from build123d import *

# Parameters (mm, degrees)
SKETCH2_R               = 18
SKETCH2_W               = 7.5
SKETCH2_H               = 7.5
BOSS_EXTRUDE1_DEPTH     = 0.9
BOSS_EXTRUDE10_START    = 0.4
SKETCH18_W              = 7.7
SKETCH18_H              = 7.7
BOSS_EXTRUDE10_DEPTH    = 0.4
BOSS_EXTRUDE2_START     = -1
SKETCH3_R               = 35
SKETCH3_R_2             = 18
BOSS_EXTRUDE2_DEPTH     = 1
SKETCH4_R               = 2.9
BOSS_EXTRUDE3_DEPTH     = 3
CUT_EXTRUDE1_DEPTH      = 50.588305073
CUT_EXTRUDE1_DEPTH_BACK = 50.588305073
SKETCH7_R               = 59.131365533
FILLET1_R               = 6


with BuildPart() as part:
    # Sketch2 → Boss-Extrude1 (new body)
    with BuildSketch(Plane.XY.offset(10)):
        Circle(SKETCH2_R)
        with BuildLine():
            Line((-8.15, -8.35), (-8.15, -14.91903147))
            ThreePointArc((-8.15, -14.91903147), (-11.939670478, -12.101415986), (-14.808021475, -8.35))
            Line((-14.808021475, -8.35), (-8.15, -8.35))
        make_face(mode=Mode.SUBTRACT)
        with BuildLine():
            Line((-8.15, -7.85), (-15.079041747, -7.85))
            ThreePointArc((-15.079041747, -7.85), (-16.470304718, -4.210589327), (-16.996396677, -0.35))
            Line((-16.996396677, -0.35), (-8.15, -0.35))
            Line((-8.15, -0.35), (-8.15, -7.85))
        make_face(mode=Mode.SUBTRACT)
        with BuildLine():
            Line((-8.15, 0.15), (-16.999338222, 0.15))
            ThreePointArc((-16.999338222, 0.15), (-16.521617742, 4.00451585), (-15.181485435, 7.65))
            Line((-15.181485435, 7.65), (-8.15, 7.65))
            Line((-8.15, 7.65), (-8.15, 0.15))
        make_face(mode=Mode.SUBTRACT)
        with BuildLine():
            Line((-8.15, 8.15), (-14.91903147, 8.15))
            ThreePointArc((-14.91903147, 8.15), (-12.02081528, 12.02081528), (-8.15, 14.91903147))
            Line((-8.15, 14.91903147), (-8.15, 8.15))
        make_face(mode=Mode.SUBTRACT)
        with BuildLine():
            Line((-7.65, 8.15), (-7.65, 15.181485435))
            ThreePointArc((-7.65, 15.181485435), (-4.00451585, 16.521617742), (-0.15, 16.999338222))
            Line((-0.15, 16.999338222), (-0.15, 8.15))
            Line((-0.15, 8.15), (-7.65, 8.15))
        make_face(mode=Mode.SUBTRACT)
        with BuildLine():
            Line((0.35, 8.15), (0.35, 16.996396677))
            ThreePointArc((0.35, 16.996396677), (4.210589327, 16.470304718), (7.85, 15.079041747))
            Line((7.85, 15.079041747), (7.85, 8.15))
            Line((7.85, 8.15), (0.35, 8.15))
        make_face(mode=Mode.SUBTRACT)
        with BuildLine():
            Line((8.35, 8.15), (8.35, 14.808021475))
            ThreePointArc((8.35, 14.808021475), (12.101415986, 11.939670478), (14.91903147, 8.15))
            Line((14.91903147, 8.15), (8.35, 8.15))
        make_face(mode=Mode.SUBTRACT)
        with BuildLine():
            Line((8.35, 7.65), (15.181485435, 7.65))
            ThreePointArc((15.181485435, 7.65), (16.521617742, 4.00451585), (16.999338222, 0.15))
            Line((16.999338222, 0.15), (8.35, 0.15))
            Line((8.35, 0.15), (8.35, 7.65))
        make_face(mode=Mode.SUBTRACT)
        with BuildLine():
            Line((8.35, -0.35), (16.996396677, -0.35))
            ThreePointArc((16.996396677, -0.35), (16.470304718, -4.210589327), (15.079041747, -7.85))
            Line((15.079041747, -7.85), (8.35, -7.85))
            Line((8.35, -7.85), (8.35, -0.35))
        make_face(mode=Mode.SUBTRACT)
        with BuildLine():
            Line((8.35, -8.35), (14.808021475, -8.35))
            ThreePointArc((14.808021475, -8.35), (12.02081528, -12.02081528), (8.35, -14.808021475))
            Line((8.35, -14.808021475), (8.35, -8.35))
        make_face(mode=Mode.SUBTRACT)
        with BuildLine():
            Line((7.85, -8.35), (7.85, -15.079041747))
            ThreePointArc((7.85, -15.079041747), (4.210589327, -16.470304718), (0.35, -16.996396677))
            Line((0.35, -16.996396677), (0.35, -8.35))
            Line((0.35, -8.35), (7.85, -8.35))
        make_face(mode=Mode.SUBTRACT)
        with BuildLine():
            Line((-0.15, -8.35), (-0.15, -16.999338222))
            ThreePointArc((-0.15, -16.999338222), (-4.00451585, -16.521617742), (-7.65, -15.181485435))
            Line((-7.65, -15.181485435), (-7.65, -8.35))
            Line((-7.65, -8.35), (-0.15, -8.35))
        make_face(mode=Mode.SUBTRACT)
        with Locations((-3.9, -4.1)):
            Rectangle(SKETCH2_W, SKETCH2_H, mode=Mode.SUBTRACT)
        with Locations((4.1, -4.1)):
            Rectangle(SKETCH2_W, SKETCH2_H, mode=Mode.SUBTRACT)
        with Locations((-3.9, 3.9)):
            Rectangle(SKETCH2_W, SKETCH2_H, mode=Mode.SUBTRACT)
        with Locations((4.1, 3.9)):
            Rectangle(SKETCH2_W, SKETCH2_H, mode=Mode.SUBTRACT)
    extrude(amount=-BOSS_EXTRUDE1_DEPTH)

    # Sketch18 → Boss-Extrude10 (add)
    with BuildSketch(Plane.XY.offset(9.1).offset(BOSS_EXTRUDE10_START)):
        with BuildLine():
            ThreePointArc((-0.15, 16.999338222), (-4.11362184, 16.494790552), (-7.85, 15.079041747))
            Line((-7.85, 15.079041747), (-7.85, 8.15))
            Line((-7.85, 8.15), (-0.15, 8.15))
            Line((-0.15, 8.15), (-0.15, 16.999338222))
        make_face()
        with Locations((4, 4)):
            Rectangle(SKETCH18_W, SKETCH18_H)
        with Locations((-4, -4)):
            Rectangle(SKETCH18_W, SKETCH18_H)
        with BuildLine():
            Line((8.15, 8.15), (14.91903147, 8.15))
            ThreePointArc((14.91903147, 8.15), (12.02081528, 12.02081528), (8.15, 14.91903147))
            Line((8.15, 14.91903147), (8.15, 8.15))
        make_face()
        with BuildLine():
            ThreePointArc((-15.079041747, 7.85), (-16.494790552, 4.11362184), (-16.999338222, 0.15))
            Line((-16.999338222, 0.15), (-8.15, 0.15))
            Line((-8.15, 0.15), (-8.15, 7.85))
            Line((-8.15, 7.85), (-15.079041747, 7.85))
        make_face()
        with BuildLine():
            Line((0.15, -8.15), (0.15, -16.999338222))
            ThreePointArc((0.15, -16.999338222), (4.11362184, -16.494790552), (7.85, -15.079041747))
            Line((7.85, -15.079041747), (7.85, -8.15))
            Line((7.85, -8.15), (0.15, -8.15))
        make_face()
        with BuildLine():
            ThreePointArc((-14.91903147, -8.15), (-12.02081528, -12.02081528), (-8.15, -14.91903147))
            Line((-8.15, -14.91903147), (-8.15, -8.15))
            Line((-8.15, -8.15), (-14.91903147, -8.15))
        make_face()
        with BuildLine():
            Line((8.15, -7.85), (15.079041747, -7.85))
            ThreePointArc((15.079041747, -7.85), (16.494790552, -4.11362184), (16.999338222, -0.15))
            Line((16.999338222, -0.15), (8.15, -0.15))
            Line((8.15, -0.15), (8.15, -7.85))
        make_face()
    extrude(amount=-BOSS_EXTRUDE10_DEPTH)

    # Sketch3 → Boss-Extrude2 (add)
    with BuildSketch(Plane(origin=(0, 0, 9.1), x_dir=(-1, 0, 0), z_dir=(0, 0, -1)).offset(BOSS_EXTRUDE2_START)):
        Circle(SKETCH3_R)
        Circle(SKETCH3_R_2, mode=Mode.SUBTRACT)
    extrude(amount=BOSS_EXTRUDE2_DEPTH)

    # Sketch4 → Boss-Extrude3 (add)
    with BuildSketch(Plane(origin=(0, 0, 9.1), x_dir=(-1, 0, 0), z_dir=(0, 0, -1))):
        with Locations((0, 29)):
            Circle(SKETCH4_R)
        with Locations((25.11473671, -14.5)):
            Circle(SKETCH4_R)
        with Locations((-25.11473671, -14.5)):
            Circle(SKETCH4_R)
    extrude(amount=-BOSS_EXTRUDE3_DEPTH)

    # Sketch7 → Cut-Extrude1 (cut, two sides: drawn at the far end of the back side and taken through both)
    with BuildSketch(Plane(origin=(0, 0, 9.1), x_dir=(-1, 0, 0), z_dir=(0, 0, -1)).offset(-CUT_EXTRUDE1_DEPTH_BACK)):
        Circle(SKETCH7_R)
        Polygon((0, 42), (-36.373066959, -21), (36.373066959, -21), align=None, mode=Mode.SUBTRACT)
    extrude(amount=CUT_EXTRUDE1_DEPTH + CUT_EXTRUDE1_DEPTH_BACK, mode=Mode.SUBTRACT)

    # Fillet1
    fillet1_edges = [part.edges().sort_by_distance(p)[0] for p in [
        (-4.186533479, 34.748711306, 9.6),
        (-32.186533479, -13.748711306, 9.6),
        (-28, -21, 9.6),
        (28, -21, 9.6),
        (32.186533479, -13.748711306, 9.6),
        (4.186533479, 34.748711306, 9.6),
    ]]
    fillet(fillet1_edges, radius=FILLET1_R)


solid = part.part
Read the model definition and answer for the solid it produces. Units are mm, in the model's axes. A direction names the side the tool comes from. Give positions to 0.01 mm unless a question says otherwise; leave off trailing zeros. Write each loop counter-clockwise with the first axis right and the second up, starting at its lowest first coordinate (ties: lowest second). Pieces come first, ordered by that corner, then holes. Notation, with made-up numbers: (12, -18) - (23, -18) arc R18 cw to (23, 16) - close; hole circle Ø5 at (60.5, 83). An arc over 180 degrees is marked (long way). Return JSON: item names as keys, results as strings.
Q1. For faces 1 (the face through (-16.457, -4.264, 9.556)), 2 (the face through (-11, -11, 9.5)), 3 (the face through (-3.67, 34.14, 9.61)), determine the directions among +Z, -Z, +X, -X, +Y, -Y from which every point of the face is accessible in a straight line to the end or side of a thin tool.
Reply:
{"face 1": "+Z, -Z", "face 2": "+Z", "face 3": "+Z, -Z, -X, +Y"}
Q2. A cutting plane is placed at B-B, the plane x = 5. Determine the outline of the cut face in (y, z).
Reply:
{"outline": "(-21, 9.1) - (-7.85, 9.1) - (-7.85, 10) - (-8.35, 10) - (-8.35, 9.5) - (-16.25, 9.5) - (-16.25, 10) - (-17.29, 10) - (-17.29, 10.1) - (-21, 10.1) - close; (-0.35, 9.1) - (8.15, 9.1) - (8.15, 10) - (7.65, 10) - (7.65, 9.5) - (0.15, 9.5) - (0.15, 10) - (-0.35, 10) - close; (16.25, 9.1) - (33.05, 9.1) - (33.05, 10.1) - (17.29, 10.1) - (17.29, 10) - (16.25, 10) - close"}
Q3. A cutting plane is placed at C-C, the plane x = 26.5. Determine the outline of the cut face in (y, z).
Reply:
{"outline": "(-20.76, 9.1) - (-3.9, 9.1) - (-3.9, 10.1) - (-11.95, 10.1) - (-11.95, 12.1) - (-17.05, 12.1) - (-17.05, 10.1) - (-20.76, 10.1) - close"}
Q4. Consider line 1 along Y through (x, z) = (0, 10.05); line 2 along Y through (x, z) = (2, 9.4); line 3 along X through (y, z) = (-8.5, 9.3). Determine where each line is inside the solid, lowest interval first. Write a range as [from, to].
Reply:
{"line 1": "[-21, -18], [18, 35]", "line 2": "[-21, -7.85], [-0.35, 8.15], [16.88, 34.82]", "line 3": "[-29.16, -7.65], [-0.15, 8.35], [14.72, 29.16]"}
Q5. Given P1, Ø12, axis at x = -9.5, y = 8.5, coming from the +Z side; P2, Ø0.7, axis at y = 12, z = 9.5, coming from the +X side; P3, Ø0.5, axis at y = 3.5, z = 9.5, coming from the +X side, each flat-ended and moving along its own axis, determine where each tip first touches the part or whether it passes through.
Reply:
{"P1": "z = 10.1", "P2": "x = 17.52", "P3": "x = 22.37"}
Q6. A cutting plane is placed at A-A, the plane y = 5.5. Determine the outline of the cut face in (x, z).
Reply:
{"outline": "(-21.07, 9.1) - (-7.65, 9.1) - (-7.65, 10) - (-8.15, 10) - (-8.15, 9.5) - (-16.09, 9.5) - (-16.09, 10) - (-17.14, 10) - (-17.14, 10.1) - (-21.07, 10.1) - close; (-0.15, 9.1) - (8.35, 9.1) - (8.35, 10) - (7.85, 10) - (7.85, 9.5) - (0.35, 9.5) - (0.35, 10) - (-0.15, 10) - close; (16.09, 9.1) - (21.07, 9.1) - (21.07, 10.1) - (17.14, 10.1) - (17.14, 10) - (16.09, 10) - close"}
Q7. For a pull along Y with two mould halves and no side action, classify faces 4 (the face through (0, 29, 12.1)), 5 (the face through (27.73, -20.247, 9.607)), 6 (the face through (4.264, -16.457, 9.754)), 7 (the face through (12.05, 11.99, 9.75)) as released by +Y, released by -Y, zero draft, split by the parting line, or undercut.
Reply:
{"face 4": "zero draft", "face 5": "released by -Y", "face 6": "undercut", "face 7": "undercut"}
